from build123d import *

# Parameters (mm, degrees)
F0_W     = 69
F0_H     = 99
F2_DEPTH = 3.5
F1_W     = 45
F1_H     = 6
F3_DEPTH = 5


with BuildPart() as f2:
    # F0 (on Top) → F2 (new body, symmetric)
    with BuildSketch(Plane.XY):
        Rectangle(F0_W, F0_H)
    extrude(amount=F2_DEPTH, both=True)

    # F1 (on face) → F3 (cut)
    with BuildSketch(Plane(origin=(0, 0, -3.5), x_dir=(1, 0, 0), z_dir=(0, 0, -1))):
        with Locations((-5, 46.5)):
            Rectangle(F1_W, F1_H)
    extrude(amount=-F3_DEPTH, mode=Mode.SUBTRACT)


solid = f2.part
Source: CAD feature listing. Evaluate the final solid. Frame: model axes, mm. A direction names the side the tool comes from. Coordinates: 2 decimals unless noted, no trailing zeros. Order: outer loops, then holes, each group sorted by start corner. A loop starts at its lowest first (then second) coordinate and runs counter-clockwise, first axis right, second up.
Item 1: Pull-direction query (X, two-part tool) for faces 1 (the face through (-34.5, -1, 0)), 2 (the face through (0, 1, 3.5)), 3 (the face through (-5, -47, 1.5)), 4 (the face through (-27.5, -46, -1)); classes: pulls with the +X half, pulls with the -X half, needs draft (parallel to the pull), parting line crosses it, or undercut.
Output values:
face 1: pulls with the -X half
face 2: needs draft
face 3: undercut
face 4: undercut
Item 2: Set-up query: faces 5 (the face through (34.5, -1, 0)), 6 (the face through (-5, -43.5, -1)). Return all of +Z, -Z, +X, -X, +Y, -Y with unobstructed straight access to the full face (end or side cutting, diameter ignored); none if empty.
Output values:
face 5: +Z, -Z, +X, +Y, -Y
face 6: -Z, -Y
Item 3: Cut plane A-A (z = -1.5). Return loops of the section in (x, y).
Output values:
outline: (-34.5, -49.5) - (-27.5, -49.5) - (-27.5, -43.5) - (17.5, -43.5) - (17.5, -49.5) - (34.5, -49.5) - (34.5, 49.5) - (-34.5, 49.5) - close
Item 4: Cut plane B-B (x = -6). Return loops of the section in (y, z).
Output values:
outline: (-49.5, 1.5) - (-43.5, 1.5) - (-43.5, -3.5) - (49.5, -3.5) - (49.5, 3.5) - (-49.5, 3.5) - close
Item 5: Material intervals for line 1 (Y direction, x = -25, z = -1.25), sorted ascending.
Output values:
line 1: y = -43.5 to 49.5
Item 6: First-contact query: P1, Ø1.8, axis at x = -11.5, y = -47.5, coming from the -Z side; P2, Ø2.5, axis at x = -1.5, z = -0.5, coming from the -Y side. Flat tips, straight axial feed; report the tip coordinate or a pass-through.
Output values:
P1: stops at z = 1.5
P2: stops at y = -43.5
